Design review of the part built by this model. Coordinates are the model's own, in mm. Give positions to 0.01 mm unless a question says otherwise; leave off trailing zeros. Write each loop counter-clockwise with the first axis right and the second up, starting at its lowest first coordinate (ties: lowest second). Pieces come first, ordered by that corner, then holes. Notation, with made-up numbers: (34.25, -38.5) -> (53.25, -38.5) arc R10 ccw to (53.25, -20.5) -> close; hole circle Ø11 at (19, -23). An arc over 180 degrees is marked (long way). Use CSV: the item, a comma, the result in double quotes.
```python
from build123d import *

# Parameters (mm, degrees)
F1_DEPTH = 100
F2_R     = 5


with BuildPart() as f1:
    # F0 (on Top) → F1 (new body)
    with BuildSketch(Plane.XY):
        with BuildLine():
            Line((40, 20), (-40, 20))
            ThreePointArc((-40, 20), (-60, 0), (-40, -20))
            Line((-40, -20), (40, -20))
            Line((40, -20), (40, 20))
        make_face()
    extrude(amount=F1_DEPTH)

    # F2
    f2_edges = [f1.edges().sort_by_distance(p)[0] for p in [
        (0, 20, 100),
        (40, 0, 100),
    ]]
    fillet(f2_edges, radius=F2_R)


solid = f1.part
```
(1) For line 1 along X through (y, z) = (9, 23); line 2 along X through (y, z) = (-4, 84.5); line 3 along Y through (x, z) = (-54.5, 62.5), list the stretches that pass through material, from the lowest coordinate up. Write a range as [from, to].
Established:
line 1,"x = [-57.86, 40]"
line 2,"x = [-59.6, 40]"
line 3,"y = [-13.77, 13.77]"
(2) Take a section at A-A (z = 50.5). Write out the cut boundary in (x, y), then the cut area to 3 significant figures.
Established:
outline,"(-40, -20) -> (40, -20) -> (40, 20) -> (-40, 20) arc R20 ccw to start"
area,"3,830 mm2"
(3) Clearance check with flat-ended pins moving along their axes: pin 1 (6 mm diameter, centred on y = -5, z = 50, fed in from -X); pin 2 (6 mm diameter, centred on y = 12.5, z = 30.5, fed in from -X); pin 3 (4 mm diameter, centred on y = -1.5, z = 26, fed in from -X). State where each tip first meets the part, or that it passes through.
Established:
pin 1,"stops at x = -59.9"
pin 2,"stops at x = -57.6"
pin 3,"stops at x = -60"
